Build history of the part. All positions in model axes, mm. Face numbers are marked on the shaded views. A direction names the side the tool comes from. Round coordinates to 2 decimals unless told otherwise and drop trailing zeros. Loops run counter-clockwise (first coordinate to the right, second up) from the corner with the lowest first, then second, coordinate; pieces in that order, holes last. Notation, with made-up numbers: (-12, -28) - (17, -28) arc R21 cw to (17, -22) - close; hole circle Ø9 at (31, 80.5). An arc over 180 degrees is marked (long way). Put each result on its own line as item: value. Start each with the question number.
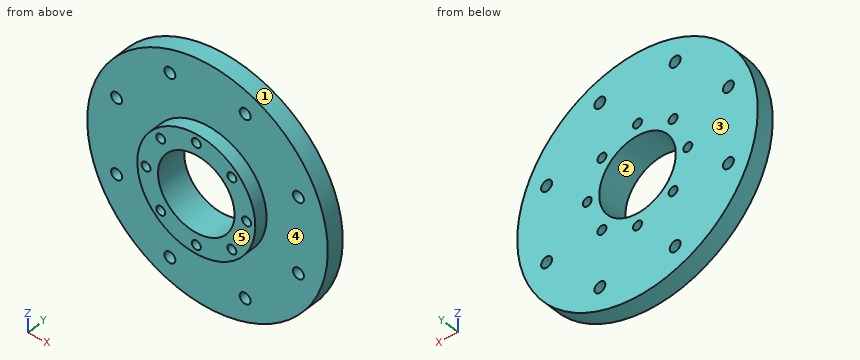
from build123d import *

# Parameters (mm, degrees)
SKETCH1_R                   = 55
BOSS_EXTRUDE1_DEPTH         = 8
SKETCH2_R                   = 27
BOSS_EXTRUDE2_DEPTH         = 6
SKETCH3_R                   = 17.5
CUT_EXTRUDE1_DEPTH          = 80.031639234
M4_CLEARANCE_HOLE1_D        = 4.1
CIRPATTERN1_COUNT           = 8
TAP_DRILL_FOR_M6X1_0_TAP1_D = 5
CIRPATTERN2_COUNT           = 8


with BuildPart() as part:
    # Sketch1 → Boss-Extrude1 (new body)
    with BuildSketch(Plane(origin=(0, 0, 0), x_dir=(1, 0, 0), z_dir=(0, 1, 0))):
        with Locations(Location((0, 0, 0), (0, 0, 270))):
            Circle(SKETCH1_R)
    extrude(amount=BOSS_EXTRUDE1_DEPTH)

    # Sketch2 → Boss-Extrude2 (add)
    with BuildSketch(Plane.XZ):
        with Locations(Location((0, 0, 0), (0, 0, 270))):
            Circle(SKETCH2_R)
    extrude(amount=BOSS_EXTRUDE2_DEPTH)

    # Sketch3 → Cut-Extrude1 (cut, through all)
    with BuildSketch(Plane(origin=(0, 8, 0), x_dir=(1, 0, 0), z_dir=(0, 1, 0))):
        with Locations(Location((0, 0, 0), (0, 0, 270))):
            Circle(SKETCH3_R)
    extrude(amount=-CUT_EXTRUDE1_DEPTH, mode=Mode.SUBTRACT)

    # M4 Clearance Hole1 (through all)
    with Locations(Plane(origin=(0, 8, 0), x_dir=(1, 0, 0), z_dir=(0, 1, 0))):
        with Locations((0, 23)):
            m4_clearance_hole1 = Hole(M4_CLEARANCE_HOLE1_D / 2)

    # CirPattern1: M4 Clearance Hole1 ×8 about axis
    cirpattern1_axis = Axis((0, 0, 0), (0, 1, 0))
    for i in range(1, CIRPATTERN1_COUNT):
        add(m4_clearance_hole1.rotate(cirpattern1_axis, i * 360 / CIRPATTERN1_COUNT), mode=Mode.SUBTRACT)

    # Tap Drill for M6x1.0 Tap1 (through all)
    with Locations(Plane(origin=(0, 8, 0), x_dir=(1, 0, 0), z_dir=(0, 1, 0))):
        with Locations((17.220754456, 41.574578963)):
            tap_drill_for_m6x1_0_tap1 = Hole(TAP_DRILL_FOR_M6X1_0_TAP1_D / 2)

    # CirPattern2: Tap Drill for M6x1.0 Tap1 ×8 about axis
    cirpattern2_axis = Axis((0, 0, 0), (0, 1, 0))
    for i in range(1, CIRPATTERN2_COUNT):
        add(tap_drill_for_m6x1_0_tap1.rotate(cirpattern2_axis, i * 360 / CIRPATTERN2_COUNT), mode=Mode.SUBTRACT)


solid = part.part
Item 1: Slice it at D-D (y = -2.25). Give the number of separate pieces and of enclosed holes in the cut face, plus the area to 3 significant figures.
Item 2: Slice it at B-B (x = -23). Give the cut face in (y, z).
Item 3: Drill centre lines: probe 1 along X at (y, z) = (0.25, -42); probe 2 along X at (y, z) = (6.75, -19); probe 3 along X at (y, z) = (-1.5, 14.5). Where is each one in solid material? Low to high. Write a range as [from, to].
Item 4: Slice it at A-A (z = 0). Give the cut face in (x, y), plus the area to 3 significant figures.
Item 5: Which spindle directions (+Z, -Z, +X, -X, +Y, -Y) get a long thin tool onto all of the face, cutting with end or side? Do the marked faces 4 and 5. Say none if no direction does.
Item 6: Drop flat-ended pins along their axis: pin 1 Ø8 at (x, y) = (-10, 1) entering from -Z; pin 2 Ø5 at (x, z) = (41, 33) entering from -Y; pin 3 Ø8 at (y, z) = (3.5, 23) entering from +X; pin 4 Ø5.5 at (x, z) = (0, 23) entering from +Y. Give the stop position or say it passes through.
Item 7: Two-plate mould, pull along Z, no slides. Class the marked faces 1, 2 and 3: pulls with the +Z half, pulls with the -Z half, needs draft (parallel to the pull), parting line crosses it, or undercut.
Item 8: Slice it at C-C (z = 23). Give the cut face in (x, y).
Computed values:
1. separate pieces: 1
1. enclosed holes: 9
1. area: 1,220 mm^2
2. outline: (-6, -14.14) - (0, -14.14) - (0, -49.96) - (8, -49.96) - (8, -2.05) - (-6, -2.05) - close; (-6, 2.05) - (8, 2.05) - (8, 49.96) - (0, 49.96) - (0, 14.14) - (-6, 14.14) - close
3. probe 1: x = [-35.51, -19.68], [-14.76, 14.76], [19.68, 35.51]
3. probe 2: x = [-51.61, -43.33], [-39.82, 39.82], [43.33, 51.61]
3. probe 3: x = [-22.78, -17.31], [-15.22, -9.8], [9.8, 15.22], [17.31, 22.78]
4. outline: (-55, 0) - (-27, 0) - (-27, -6) - (-25.05, -6) - (-25.05, 8) - (-55, 8) - close; (-20.95, -6) - (-17.5, -6) - (-17.5, 8) - (-20.95, 8) - close; (17.5, -6) - (20.95, -6) - (20.95, 8) - (17.5, 8) - close; (25.05, -6) - (27, -6) - (27, 0) - (55, 0) - (55, 8) - (25.05, 8) - close
4. area: 599 mm^2
5. face 4: -Y
5. face 5: +Z, -Z, +X, -X, -Y
6. pin 1: stops at z = -54.67
6. pin 2: stops at y = 0
6. pin 3: stops at x = 51.61
6. pin 4: stops at y = 8
7. face 1: parting line crosses it
7. face 2: undercut
7. face 3: needs draft
8. outline: (-49.96, 0) - (-14.14, 0) - (-14.14, -6) - (-2.05, -6) - (-2.05, 8) - (-49.96, 8) - close; (2.05, -6) - (14.14, -6) - (14.14, 0) - (49.96, 0) - (49.96, 8) - (2.05, 8) - close
